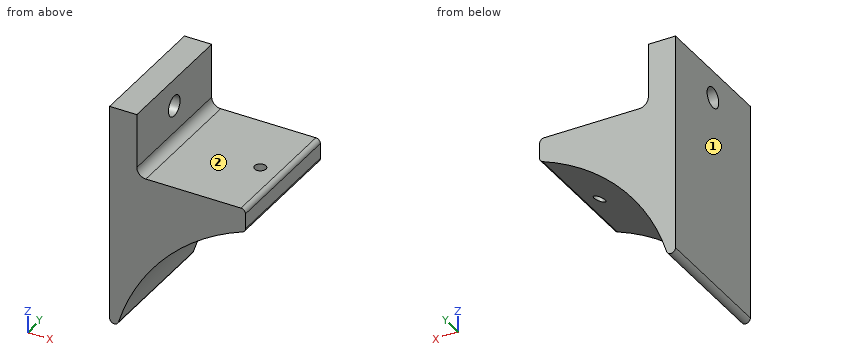
from build123d import *

# Parameters (mm, degrees)
BOSS_EXTRUDE1_DEPTH     = 14.5
SKETCH2_R               = 2.25
CUT_EXTRUDE1_DEPTH      = 68.590679831
CUT_EXTRUDE2_DEPTH      = 59.873665056
CUT_EXTRUDE2_DEPTH_BACK = 59.873665056
SKETCH3_R               = 1.25


with BuildPart() as part:
    # Sketch1 → Boss-Extrude1 (new, symmetric)
    with BuildSketch(Plane(origin=(0, 0, 0), x_dir=(1, 0, 0), z_dir=(0, 1, 0))):
        with BuildLine():
            Line((-45, -13.416407865), (-45, -61.5))
            Line((-45, -61.5), (-39, -61.5))
            Line((-39, -61.5), (-39, -49.5))
            ThreePointArc((-39, -49.5), (-38.414213562, -48.085786438), (-37, -47.5))
            Line((-37, -47.5), (-16, -47.5))
            ThreePointArc((-16, -47.5), (-15.292893219, -47.207106781), (-15, -46.5))
            Line((-15, -46.5), (-15, -43.127717306))
            ThreePointArc((-15, -43.127717306), (-15.179077931, -42.556677065), (-15.652173913, -42.190158234))
            ThreePointArc((-15.652173913, -42.190158234), (-32.748960764, -30.862688944), (-43.043478261, -13.124746824))
            ThreePointArc((-43.043478261, -13.124746824), (-44.147441956, -12.427337155), (-45, -13.416407865))
        make_face()
    extrude(amount=BOSS_EXTRUDE1_DEPTH, both=True)

    # Sketch2 → Cut-Extrude1 (cut, through all)
    with BuildSketch(Plane(origin=(-39, 0, 0), x_dir=(0, 0, -1), z_dir=(1, 0, 0))):
        with Locations((-55.5, 0)):
            Circle(SKETCH2_R)
    extrude(amount=-CUT_EXTRUDE1_DEPTH, mode=Mode.SUBTRACT)

    # Sketch3 → Cut-Extrude2 (cut, two sides: drawn at the far end of the back side and taken through both)
    with BuildSketch(Plane.XY.offset(47.5).offset(-CUT_EXTRUDE2_DEPTH_BACK)):
        with Locations((-20, 0)):
            Circle(SKETCH3_R)
    extrude(amount=CUT_EXTRUDE2_DEPTH + CUT_EXTRUDE2_DEPTH_BACK, mode=Mode.SUBTRACT)


solid = part.part
Verification items for the finished model (mm, model axes). Face numbers are marked on the shaded views. A direction names the side the tool comes from. Round coordinates to 2 decimals unless told otherwise and drop trailing zeros. Loops run counter-clockwise (first coordinate to the right, second up) from the corner with the lowest first, then second, coordinate; pieces in that order, holes last. Notation, with made-up numbers: (61, 38.5) - (94, 38.5) arc R26 ccw to (94, 56.5) - close; hole circle Ø11 at (-17, -13). An arc over 180 degrees is marked (long way). Use a Markdown table: item, result. Add a question column.
1. Section check A-A, the plane z = 55.5. Record the boundary of the cut face in (x, y).
2. Section check B-B, the plane y = -6.75. Record the boundary of the cut face in (x, z), plus the area to 3 significant figures.
3. Gauge pin test, flat ends, axial feed: pin 1 (8 mm diameter, centred on x = -24.5, y = -4, fed in from -Z); pin 2 (1 mm diameter, centred on x = -37.5, y = -2.5, fed in from +Z); pin 3 (1 mm diameter, centred on y = 1.5, z = 23, fed in from +X). Record the tip position at first contact, or that the pin passes through.
4. Access from +Z, -Z, +X, -X, +Y, -Y to the whole of each face (thin tool, end or side, straight path). Record for the marked faces 1 and 2.
5. Section check D-D, the plane y = 0. Record the boundary of the cut face in (x, z).
6. Section check C-C, the plane x = -20. Record the boundary of the cut face in (y, z).
7. Thickness scan on probe 1 along Y at (x, z) = (-20, 42); probe 2 along X at (y, z) = (0, 43.5); probe 3 along Y at (x, z) = (-40.15, 55.5). Record the ranges inside material, lowest first. Write a range as [from, to].
Checks:
| question | item | result |
|---|---|---|
| 1 | outline | (-45, -14.5) - (-39, -14.5) - (-39, -2.25) - (-45, -2.25) - close; (-45, 2.25) - (-39, 2.25) - (-39, 14.5) - (-45, 14.5) - close |
| 2 | outline | (-45, 13.42) arc R1 ccw to (-43.04, 13.12) arc R45 cw to (-15.65, 42.19) arc R1 ccw to (-15, 43.13) - (-15, 46.5) arc R1 ccw to (-16, 47.5) - (-37, 47.5) arc R2 cw to (-39, 49.5) - (-39, 61.5) - (-45, 61.5) - close |
| 2 | area | 574 mm^2 |
| 3 | pin 1 | stops at z = 34.82 |
| 3 | pin 2 | stops at z = 47.77 |
| 3 | pin 3 | stops at x = -38.38 |
| 4 | face 1 | +Z, -Z, -X, +Y, -Y |
| 4 | face 2 | +Z, +X, +Y, -Y |
| 5 | outline | (-45, 13.42) arc R1 ccw to (-43.04, 13.12) arc R45 cw to (-21.25, 39.67) - (-21.25, 47.5) - (-37, 47.5) arc R2 cw to (-39, 49.5) - (-39, 53.25) - (-45, 53.25) - close; (-45, 57.75) - (-39, 57.75) - (-39, 61.5) - (-45, 61.5) - close; (-18.75, 40.91) arc R45 cw to (-15.65, 42.19) arc R1 ccw to (-15, 43.13) - (-15, 46.5) arc R1 ccw to (-16, 47.5) - (-18.75, 47.5) - close |
| 6 | outline | (-14.5, 40.31) - (-1.25, 40.31) - (-1.25, 47.5) - (-14.5, 47.5) - close; (1.25, 40.31) - (14.5, 40.31) - (14.5, 47.5) - (1.25, 47.5) - close |
| 7 | probe 1 | y = [-14.5, -1.25], [1.25, 14.5] |
| 7 | probe 2 | x = [-45, -21.25], [-18.75, -15] |
| 7 | probe 3 | y = [-14.5, -2.25], [2.25, 14.5] |
